Geometry check sheet. Reference: the model listing, model coordinates, mm. A direction names the side the tool comes from. Round coordinates to 2 decimals unless told otherwise and drop trailing zeros. Loops run counter-clockwise (first coordinate to the right, second up) from the corner with the lowest first, then second, coordinate; pieces in that order, holes last.
```python
from build123d import *

# Parameters (mm, degrees)
SKETCH3_R          = 15
CUT_EXTRUDE1_DEPTH = 10
CUT_EXTRUDE1_DRAFT = -15


with BuildPart() as part:
    # Sketch1 → Revolve1 (revolve)
    with BuildSketch(Plane.XY, mode=Mode.PRIVATE) as revolve1_sk:
        with BuildLine():
            Line((0, 0), (0, 220))
            Line((0, 220), (20, 220))
            ThreePointArc((20, 220), (30, 210), (20, 200))
            Line((20, 200), (20, 160))
            ThreePointArc((20, 160), (40, 140), (20, 120))
            Line((20, 120), (20, 80))
            ThreePointArc((20, 80), (37.573593129, 37.573593129), (80, 20))
            ThreePointArc((80, 20), (87.360679775, 11.180339887), (90, 0))
            Line((90, 0), (0, 0))
        make_face()
    revolve(revolve1_sk.sketch.rotate(Axis((0, 0, 0), (0, 1, 0)), 90), axis=Axis((0, 0, 0), (0, 1, 0)))


with BuildPart() as cut_extrude1_tool:
    # Sketch3 → Cut-Extrude1 (with draft: the straight prism first)
    with BuildSketch(Plane(origin=(0, 220, 0), x_dir=(1, 0, 0), z_dir=(0, 1, 0))):
        Circle(SKETCH3_R)
    extrude(amount=-CUT_EXTRUDE1_DEPTH)
    # Cut-Extrude1: the draft: its side faces are tilted about the plane it starts from
    cut_extrude1_sides = [cut_extrude1_tool.faces().sort_by_distance(p)[0] for p in [
        (-15, 215, 0),
    ]]
    draft(cut_extrude1_sides, Plane(origin=(0, 220, 0), x_dir=(1, 0, 0), z_dir=(0, 1, 0)), CUT_EXTRUDE1_DRAFT)


with BuildPart() as part_1:
    add(part.part)

    # Cut-Extrude1: cut by cut_extrude1_tool
    add(cut_extrude1_tool.part, mode=Mode.SUBTRACT)


solid = part_1.part
```
1) Sectioned sample at B-B, the plane x = 26.5. State how many separate pieces and enclosed holes the cut face has, then the cut area to 3 significant figures.
Report:
separate pieces: 3
enclosed holes: 0
area: 7,490 mm2
2) Scan lines: line 1 along Y through (x, z) = (3, 11); line 2 along Y through (x, z) = (13.5, 77); line 3 along X through (y, z) = (177, -1.5). Record each from-to range of solid material in increasing order.
Report:
line 1: y = 0 to 210
line 2: y = 0 to 20.03
line 3: x = -19.94 to 19.94
3) Access from +Z, -Z, +X, -X, +Y, -Y to the whole of each face (thin tool, end or side, straight path). Record for faces 4 (the face through (-0.88, 179.72, 19.98)), 5 (the face through (-10.15, 211.74, 7.78)).
Report:
face 4: none
face 5: +Y
4) Sectioned sample at C-C, the plane y = 30.5. Record the cut outline in (x, z).
Report:
outline: circle Ø92.18 at (0, 0)
5) Gauge pin test, flat ends, axial feed: pin 1 (12 mm diameter, centred on y = 138.5, z = 10, fed in from +X); pin 2 (12 mm diameter, centred on x = -11.5, y = 40.5, fed in from +Z). Record the tip position at first contact, or that the pin passes through.
Report:
pin 1: stops at x = 39.79
pin 2: stops at z = 39.42
6) Mould release check, pull along Y, two halves, no side actions. Record for faces 1 (the face through (0, 210, 0)), 2 (the face through (-0.88, 99.72, 19.98)), 3 (the face through (-1, 0, 1)): +Y half, -Y half, draft (parallel to the pull), parting line (faces both ways), or undercut.
Report:
face 1: +Y half
face 2: undercut
face 3: -Y half
7) Sectioned sample at A-A, the plane y = 90.5. Record the cut outline in (x, z), then the cut area to 3 significant figures.
Report:
outline: circle Ø40 at (0, 0)
area: 1,260 mm2
